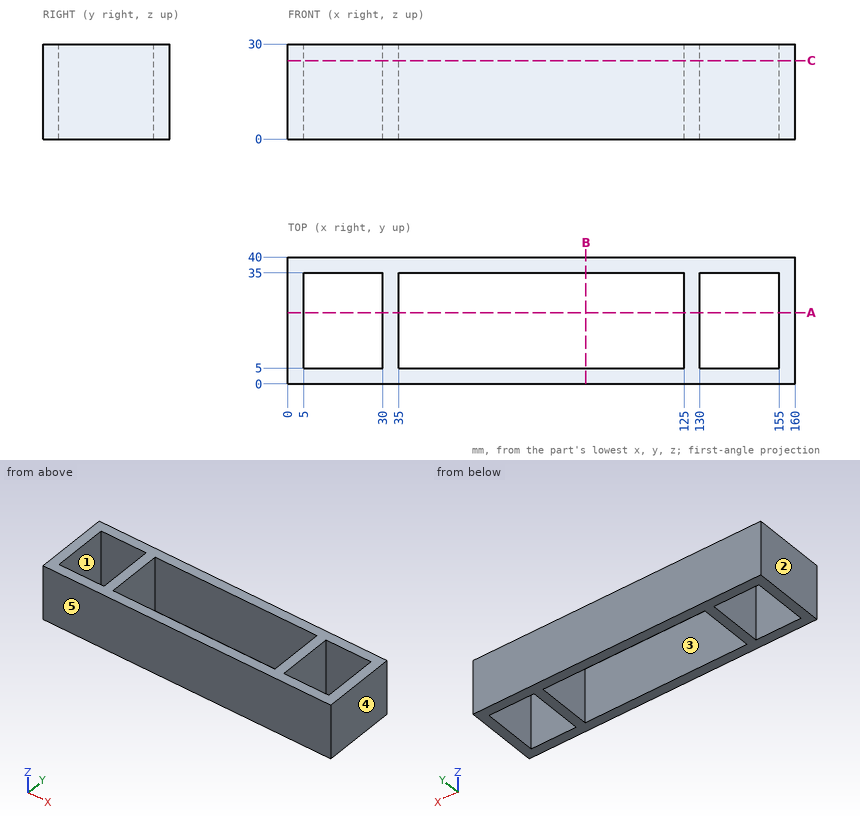
Can you work these out from the drawing? Everything is in mm from the part's minimum corner. A direction names the side the tool comes from. Round coordinates to 2 decimals unless told otherwise and drop trailing zeros. Write each loop counter-clockwise with the first axis right and the second up, starting at its lowest first coordinate (ties: lowest second). Pieces come first, ordered by that corner, then holes. Notation, with made-up numbers: M -27.5,-17 L 3.5,-17 A19 ccw 3.5,-2 Z; hole C 21,22 d9. An arc over 180 degrees is marked long. Use a Markdown table: item, result.
Item 1: We'd pull the mould along Y, two halves only. Please class the marked faces 3, 4 and 5: released by +Y, released by -Y, zero draft, split by the parting line, or undercut.
Found:
| item | result |
|---|---|
| face 3 | undercut |
| face 4 | zero draft |
| face 5 | released by -Y |
Item 2: I want a section at A-A (y = 22.5). List the corners of the cut face in (x, z) for me.
Found:
| item | result |
|---|---|
| outline | M 0,0 L 5,0 L 5,30 L 0,30 Z; M 30,0 L 35,0 L 35,30 L 30,30 Z; M 125,0 L 130,0 L 130,30 L 125,30 Z; M 155,0 L 160,0 L 160,30 L 155,30 Z |
Item 3: Which directions (+Z, -Z, +X, -X, +Y, -Y) give clear straight access to the entire face, cutting with the end or side of a thin tool? Please do the marked faces 1 and 2.
Found:
| item | result |
|---|---|
| face 1 | +Z, -Z |
| face 2 | +Z, -Z, -X, +Y, -Y |
Item 4: I want a section at B-B (x = 94). List the corners of the cut face in (y, z) for me, and give its area (3 significant figures).
Found:
| item | result |
|---|---|
| outline | M 0,0 L 5,0 L 5,30 L 0,30 Z; M 35,0 L 40,0 L 40,30 L 35,30 Z |
| area | 300 mm2 |
Item 5: I want a section at C-C (z = 24.75). List the corners of the cut face in (x, y) for me.
Found:
| item | result |
|---|---|
| outline | M 0,0 L 160,0 L 160,40 L 0,40 Z; hole M 5,5 L 30,5 L 30,35 L 5,35 Z; hole M 35,5 L 125,5 L 125,35 L 35,35 Z; hole M 130,5 L 155,5 L 155,35 L 130,35 Z |
Item 6: If I drill on line 1 along X through (y, z) = (9, 2); line 2 along Y through (x, z) = (108, 15), over which ranges is the centre line in solid material (lowest first)? Write a range as [from, to].
Found:
| item | result |
|---|---|
| line 1 | x = [0, 5], [30, 35], [125, 130], [155, 160] |
| line 2 | y = [0, 5], [35, 40] |
